```python
from build123d import *

# Parameters (mm, degrees)
F0_W     = 125
F0_H     = 2234
F1_DEPTH = 100
F3_DEPTH = 100.001


with BuildPart() as f1:
    # F0 (on Front) → F1 (new body)
    with BuildSketch(Plane.XZ):
        Polygon((-582, 0), (0, 0), (0, 125), (-125, 125), (-457, 125), (-582, 125), align=None)
        with Locations((-62.5, 1242)):
            Rectangle(F0_W, F0_H)
        with Locations((-519.5, 1242)):
            Rectangle(F0_W, F0_H)
        Polygon((-125, 2359), (0, 2359), (0, 2484), (-582, 2484), (-582, 2359), (-457, 2359), align=None)
    extrude(amount=F1_DEPTH)

    # F2 (on face) → F3 (cut, through all)
    with BuildSketch(Plane(origin=(0, 0, 0), x_dir=(-1, 0, 0), z_dir=(0, 1, 0))):
        with BuildLine():
            ThreePointArc((291, 2433.5), (283.575379, 2415.575379), (301.5, 2423))
            ThreePointArc((301.5, 2423), (298.424621, 2430.424621), (291, 2433.5))
        make_face()
        with BuildLine():
            ThreePointArc((291, 50.5), (298.424621, 53.575379), (301.5, 61))
            ThreePointArc((301.5, 61), (283.575379, 68.424621), (291, 50.5))
        make_face()
    extrude(amount=-F3_DEPTH, mode=Mode.SUBTRACT)


solid = f1.part
```
Input: part model. Units: mm. Frame: model coordinates. A direction names the side the tool comes from. Round coordinates to 2 decimals unless told otherwise and drop trailing zeros. Write each loop counter-clockwise with the first axis right and the second up, starting at its lowest first coordinate (ties: lowest second). Pieces come first, ordered by that corner, then holes. Notation, with made-up numbers: (33.5, 32.5) -> (67.5, 32.5) arc R9 ccw to (67.5, 49.5) -> close; hole circle Ø9 at (4, -15). An arc over 180 degrees is marked (long way). Answer as CSV lines item,"result".
1. Reachability of faces 5 (the flat face through (-293, -49, 2359)), 6 (the flat face through (-101, 0, 1259)) from +Z, -Z, +X, -X, +Y, -Y: full face, straight path, thin tool, end or side. Return the list, or none.
Geometry says:
face 5,"+Y, -Y"
face 6,"+Z, -Z, +X, -X, +Y"
2. Ray query, L1, parallel to Z at x = -291, y = -59; L2, parallel to X at y = -56, z = 342.5; L3, parallel to Z at x = -132.5, y = -53. Return the intervals inside material, ascending. Write a range as [from, to].
Geometry says:
L1,"z = [0, 50.5], [71.5, 125], [2359, 2412.5], [2433.5, 2484]"
L2,"x = [-582, -457], [-125, 0]"
L3,"z = [0, 125], [2359, 2484]"
3. Mould query, pull axis X, two halves, no side actions, for faces 1 (the flat face through (0, -49, 1225)), 2 (the flat face through (-582, -49, 1259)), 3 (the flat face through (-101, -100, 1259)), 4 (the flat face through (-125, -49, 1226)). Classes: +X half, -X half, draft (parallel to the pull), parting line (faces both ways), or undercut.
Geometry says:
face 1,"+X half"
face 2,"-X half"
face 3,"draft"
face 4,"undercut"
4. Section C-C (y = -78.5). Return the cut outline in (x, z), plus the area to 3 significant figures.
Geometry says:
outline,"(-582, 0) -> (0, 0) -> (0, 2484) -> (-582, 2484) -> close; hole (-457, 125) -> (-125, 125) -> (-125, 2359) -> (-457, 2359) -> close; hole circle Ø21 at (-291, 61); hole circle Ø21 at (-291, 2423)"
area,"703,000 mm^2"
5. Section B-B (x = -354.5). Return the cut outline in (y, z).
Geometry says:
outline,"(-100, 0) -> (0, 0) -> (0, 125) -> (-100, 125) -> close; (-100, 2359) -> (0, 2359) -> (0, 2484) -> (-100, 2484) -> close"
6. Section A-A (z = 417). Return the cut outline in (x, y), plus the area to 3 significant figures.
Geometry says:
outline,"(-582, -100) -> (-457, -100) -> (-457, 0) -> (-582, 0) -> close; (-125, -100) -> (0, -100) -> (0, 0) -> (-125, 0) -> close"
area,"25,000 mm^2"
